Design review of the part built by this model. Coordinates are the model's own, in mm. Face numbers are marked on the shaded views. A direction names the side the tool comes from. Coordinates: 2 decimals unless noted, no trailing zeros. Loops run counter-clockwise (first coordinate to the right, second up) from the corner with the lowest first, then second, coordinate; pieces in that order, holes last. Notation, with made-up numbers: (39.5, -39.5) - (62.5, -39.5) arc R30 cw to (62.5, -0.5) - close; hole circle Ø2 at (-30.75, 88). An arc over 180 degrees is marked (long way). Use one line per item in the form item = value. Start each with the question number.
(1) Tool access review of the marked faces 4, 5 and 6: name each direction out of +Z, -Z, +X, -X, +Y, -Y from which nothing blocks a thin tool from reaching the whole face with its end or side.
(2) Add section C-C (z = -8). State the section outline as (x, y) points.
(3) Clearance check with flat-ended pins moving along their axes: pin 1 Ø13 at (x, z) = (26, -27) entering from +Y; pin 2 Ø4.5 at (x, z) = (-29, -8) entering from +Y (3 decimals); pin 3 Ø3.5 at (y, z) = (19.5, -33.5) entering from +X; pin 4 Ø5.5 at (y, z) = (20.5, -34.5) entering from -X. State where each tip first meets the part, or that it passes through.
(4) Add section D-D (y = 6). State the section outline as (x, z) points.
(5) For L1, parallel to X at y = 3, z = -29; L2, parallel to Z at x = -29, y = 2.85; L3, parallel to Y at x = 0, z = -7.5, list the stretches that pass through material, from the lowest coordinate up.
(6) Add section B-B (z = -30). State the section outline as (x, y) points.
(7) The part is to be moulded in two halves that separate along X. For the marked faces 1, 2 and 3, say which applies: pulls with the +X half, pulls with the -X half, needs draft (parallel to the pull), parting line crosses it, or undercut.
(8) Add section A-A (x = -25). State the section outline as (y, z) points.
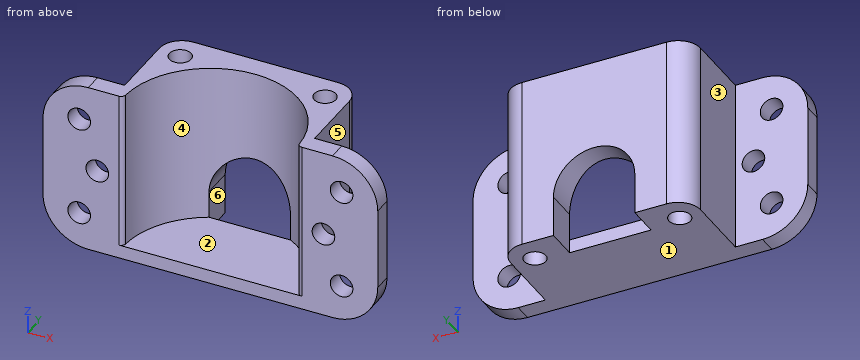
```python
from build123d import *

# Parameters (mm, degrees)
SKETCH1_W           = 42
SKETCH1_H           = 48
SKETCH1_R           = 19.25
SKETCH1_R_2         = 2.4
BOSS_EXTRUDE1_DEPTH = 35
SKETCH4_W           = 19
SKETCH4_H           = 5
BOSS_EXTRUDE3_DEPTH = 35
CUT_EXTRUDE1_REACH  = 70.367
SKETCH5_R           = 2.5
BOSS_EXTRUDE4_DEPTH = 3
CUT_EXTRUDE2_REACH  = 62.166
SKETCH9_W           = 16
SKETCH9_H           = 4
BOSS_EXTRUDE6_DEPTH = 38
CUT_EXTRUDE3_REACH  = 58.683
SKETCH10_R          = 2.5
FILLET1_R           = 10
FILLET2_R           = 5
SKETCH11_R          = 2.4
CUT_EXTRUDE4_DEPTH  = 57.302753041
FILLET3_R           = 1
CUT_EXTRUDE7_DEPTH  = 7


with BuildPart() as part:
    # Sketch1 → Boss-Extrude1 (new body)
    with BuildSketch(Plane.XY):
        Rectangle(SKETCH1_W, SKETCH1_H)
        Circle(SKETCH1_R, mode=Mode.SUBTRACT)
        with Locations((-16, 18.285714286)):
            Circle(SKETCH1_R_2, mode=Mode.SUBTRACT)
        with Locations((16, 18.285714286)):
            Circle(SKETCH1_R_2, mode=Mode.SUBTRACT)
        with Locations((16, -18.285714286)):
            Circle(SKETCH1_R_2, mode=Mode.SUBTRACT)
        with Locations((-16, -18.285714286)):
            Circle(SKETCH1_R_2, mode=Mode.SUBTRACT)
    extrude(amount=-BOSS_EXTRUDE1_DEPTH)

    # Sketch4 → Boss-Extrude3 (add)
    with BuildSketch(Plane.XY):
        with Locations((-30.5, -21.5)):
            Rectangle(SKETCH4_W, SKETCH4_H)
        with Locations((30.5, -21.5)):
            Rectangle(SKETCH4_W, SKETCH4_H)
    extrude(amount=-BOSS_EXTRUDE3_DEPTH)

    # Sketch5 → Cut-Extrude1 (cut, up to next)
    with BuildSketch(Plane(origin=(0, -19, 0), x_dir=(1, 0, 0), z_dir=(0, 1, 0)), mode=Mode.PRIVATE) as cut_extrude1_sk1:
        with Locations(Location((-25, 19, 0), (0, 0, 270))):
            Circle(SKETCH5_R)
    cut_extrude1_tool1 = extrude(cut_extrude1_sk1.sketch, amount=-CUT_EXTRUDE1_REACH, mode=Mode.PRIVATE) & part.part
    # Sketch5 → Cut-Extrude1 (cut, up to next)
    with BuildSketch(Plane(origin=(0, -19, 0), x_dir=(1, 0, 0), z_dir=(0, 1, 0)), mode=Mode.PRIVATE) as cut_extrude1_sk2:
        with Locations(Location((25, 19, 0), (0, 0, 270))):
            Circle(SKETCH5_R)
    cut_extrude1_tool2 = extrude(cut_extrude1_sk2.sketch, amount=-CUT_EXTRUDE1_REACH, mode=Mode.PRIVATE) & part.part
    add(cut_extrude1_tool1.solids().sort_by_distance((-25, -19, -19))[0], mode=Mode.SUBTRACT)
    add(cut_extrude1_tool2.solids().sort_by_distance((25, -19, -19))[0], mode=Mode.SUBTRACT)

    # Sketch6 → Boss-Extrude4 (add)
    with BuildSketch(Plane(origin=(0, 0, -35), x_dir=(-1, 0, 0), z_dir=(0, 0, -1))):
        Polygon((-21, 24), (-21, -19), (-40, -19), (-40, -24), (40, -24), (40, -19), (21, -19), (21, 24), align=None)
    extrude(amount=BOSS_EXTRUDE4_DEPTH)

    # Sketch7 → Cut-Extrude2 (cut, up to next)
    with BuildSketch(Plane.XY, mode=Mode.PRIVATE) as cut_extrude2_sk1:
        Polygon((-21, 0), (21, 0), (21, -19), (40, -19), (40, -24), (-40, -24), (-40, -19), (-21, -19), align=None)
    cut_extrude2_tool1 = extrude(cut_extrude2_sk1.sketch, amount=-CUT_EXTRUDE2_REACH, mode=Mode.PRIVATE) & part.part
    add(cut_extrude2_tool1.solids().sort_by_distance((0, -13.506678, 0))[0], mode=Mode.SUBTRACT)

    # Sketch9 → Boss-Extrude6 (add)
    with BuildSketch(Plane.XY):
        with Locations((-29, 2)):
            Rectangle(SKETCH9_W, SKETCH9_H)
        with Locations((29, 2)):
            Rectangle(SKETCH9_W, SKETCH9_H)
    extrude(amount=-BOSS_EXTRUDE6_DEPTH)

    # Sketch10 → Cut-Extrude3 (cut, up to next)
    with BuildSketch(Plane(origin=(0, 4, 0), x_dir=(1, 0, 0), z_dir=(0, 1, 0)), mode=Mode.PRIVATE) as cut_extrude3_sk1:
        with Locations(Location((-29, 8, 0), (0, 0, 180))):
            Circle(SKETCH10_R)
    cut_extrude3_tool1 = extrude(cut_extrude3_sk1.sketch, amount=-CUT_EXTRUDE3_REACH, mode=Mode.PRIVATE) & part.part
    # Sketch10 → Cut-Extrude3 (cut, up to next)
    with BuildSketch(Plane(origin=(0, 4, 0), x_dir=(1, 0, 0), z_dir=(0, 1, 0)), mode=Mode.PRIVATE) as cut_extrude3_sk2:
        with Locations(Location((-29, 30, 0), (0, 0, 180))):
            Circle(SKETCH10_R)
    cut_extrude3_tool2 = extrude(cut_extrude3_sk2.sketch, amount=-CUT_EXTRUDE3_REACH, mode=Mode.PRIVATE) & part.part
    # Sketch10 → Cut-Extrude3 (cut, up to next)
    with BuildSketch(Plane(origin=(0, 4, 0), x_dir=(1, 0, 0), z_dir=(0, 1, 0)), mode=Mode.PRIVATE) as cut_extrude3_sk3:
        with Locations(Location((29, 30, 0), (0, 0, 270))):
            Circle(SKETCH10_R)
    cut_extrude3_tool3 = extrude(cut_extrude3_sk3.sketch, amount=-CUT_EXTRUDE3_REACH, mode=Mode.PRIVATE) & part.part
    # Sketch10 → Cut-Extrude3 (cut, up to next)
    with BuildSketch(Plane(origin=(0, 4, 0), x_dir=(1, 0, 0), z_dir=(0, 1, 0)), mode=Mode.PRIVATE) as cut_extrude3_sk4:
        with Locations(Location((29, 8, 0), (0, 0, 270))):
            Circle(SKETCH10_R)
    cut_extrude3_tool4 = extrude(cut_extrude3_sk4.sketch, amount=-CUT_EXTRUDE3_REACH, mode=Mode.PRIVATE) & part.part
    # Sketch10 → Cut-Extrude3 (cut, up to next)
    with BuildSketch(Plane(origin=(0, 4, 0), x_dir=(1, 0, 0), z_dir=(0, 1, 0)), mode=Mode.PRIVATE) as cut_extrude3_sk5:
        with Locations(Location((-25, 19, 0), (0, 0, 180))):
            Circle(SKETCH10_R)
    cut_extrude3_tool5 = extrude(cut_extrude3_sk5.sketch, amount=-CUT_EXTRUDE3_REACH, mode=Mode.PRIVATE) & part.part
    # Sketch10 → Cut-Extrude3 (cut, up to next)
    with BuildSketch(Plane(origin=(0, 4, 0), x_dir=(1, 0, 0), z_dir=(0, 1, 0)), mode=Mode.PRIVATE) as cut_extrude3_sk6:
        with Locations(Location((25, 19, 0), (0, 0, 270))):
            Circle(SKETCH10_R)
    cut_extrude3_tool6 = extrude(cut_extrude3_sk6.sketch, amount=-CUT_EXTRUDE3_REACH, mode=Mode.PRIVATE) & part.part
    add(cut_extrude3_tool1.solids().sort_by_distance((-29, 4, -8))[0], mode=Mode.SUBTRACT)
    add(cut_extrude3_tool2.solids().sort_by_distance((-29, 4, -30))[0], mode=Mode.SUBTRACT)
    add(cut_extrude3_tool3.solids().sort_by_distance((29, 4, -30))[0], mode=Mode.SUBTRACT)
    add(cut_extrude3_tool4.solids().sort_by_distance((29, 4, -8))[0], mode=Mode.SUBTRACT)
    add(cut_extrude3_tool5.solids().sort_by_distance((-25, 4, -19))[0], mode=Mode.SUBTRACT)
    add(cut_extrude3_tool6.solids().sort_by_distance((25, 4, -19))[0], mode=Mode.SUBTRACT)

    # Fillet1
    fillet1_edges = [part.edges().sort_by_distance(p)[0] for p in [
        (-37, 2, 0),
        (-37, 2, -38),
        (37, 2, 0),
        (37, 2, -38),
    ]]
    fillet(fillet1_edges, radius=FILLET1_R)

    # Fillet2
    fillet2_edges = [part.edges().sort_by_distance(p)[0] for p in [
        (-21, 24, -19),
        (21, 24, -19),
    ]]
    fillet(fillet2_edges, radius=FILLET2_R)

    # Sketch11 → Cut-Extrude4 (cut, through all)
    with BuildSketch(Plane.XY.offset(-35)):
        with Locations((16, 18.285714286)):
            Circle(SKETCH11_R)
        with Locations((-16, 18.285714286)):
            Circle(SKETCH11_R)
    extrude(amount=-CUT_EXTRUDE4_DEPTH, mode=Mode.SUBTRACT)

    # Fillet3
    fillet3_edges = [part.edges().sort_by_distance(p)[0] for p in [
        (-19.25, 0, -17.5),
        (19.25, 0, -17.5),
    ]]
    fillet(fillet3_edges, radius=FILLET3_R)

    # Sketch12 → Cut-Extrude7 (cut)
    with BuildSketch(Plane(origin=(0, 24, 0), x_dir=(1, 0, 0), z_dir=(0, 1, 0))):
        with BuildLine():
            ThreePointArc((1.6e-08, 38), (-6.363961025, 35.363961036), (-9, 29))
            Line((-9, 29), (9, 29))
            ThreePointArc((9, 29), (6.363961036, 35.363961025), (1.6e-08, 38))
        make_face()
        with BuildLine():
            Line((9, 29), (-9, 29))
            ThreePointArc((-9, 29), (0, 20), (9, 29))
        make_face()
        with BuildLine():
            ThreePointArc((1.6e-08, 38), (6.363961036, 35.363961025), (9, 29))
            Line((9, 29), (9, 38))
            Line((9, 38), (1.6e-08, 38))
        make_face()
        with BuildLine():
            Line((-9, 38), (-9, 29))
            ThreePointArc((-9, 29), (-6.363961025, 35.363961036), (1.6e-08, 38))
            Line((1.6e-08, 38), (-9, 38))
        make_face()
    extrude(amount=-CUT_EXTRUDE7_DEPTH, mode=Mode.SUBTRACT)


solid = part.part
```
Computed values:
q1.face_4 = +Z, -Y
q1.face_5 = +Z, -Z, +X, +Y
q1.face_6 = -Z, +Y
q2.outline = (-36.8, 0) - (-31.5, 0) - (-31.5, 4) - (-36.8, 4) - close; (-26.5, 0) - (-20.23, 0) arc R1 ccw to (-19.23, 0.95) arc R19.25 cw to (19.23, 0.95) arc R1 ccw to (20.23, 0) - (26.5, 0) - (26.5, 4) - (21, 4) - (21, 19) arc R5 ccw to (16, 24) - (-16, 24) arc R5 ccw to (-21, 19) - (-21, 4) - (-26.5, 4) - close; (31.5, 0) - (36.8, 0) - (36.8, 4) - (31.5, 4) - close; hole circle Ø4.8 at (-16, 18.29); hole circle Ø4.8 at (16, 18.29)
q3.pin_1 = 22.57
q3.pin_2 = through
q3.pin_3 = 21
q3.pin_4 = -21
q4.outline = (-21, -38) - (21, -38) - (21, 0) - (18.29, 0) - (18.29, -35) - (-18.29, -35) - (-18.29, 0) - (-21, 0) - close
q5.L1 = -36.95 to -31.29, -26.71 to -19.01, 19.01 to 26.71, 31.29 to 36.95
q5.L2 = -37.8 to -32.5, -27.5 to -10.5, -5.5 to -0.2
q5.L3 = 19.25 to 24
q6.outline = (-36.8, 0) - (-31.5, 0) - (-31.5, 4) - (-36.8, 4) - close; (-26.5, 0) - (-20.23, 0) arc R1 ccw to (-19.23, 0.95) arc R19.25 cw to (-9, 17.02) - (-9, 24) - (-16, 24) arc R5 ccw to (-21, 19) - (-21, 4) - (-26.5, 4) - close; (9, 17.02) arc R19.25 cw to (19.23, 0.95) arc R1 ccw to (20.23, 0) - (26.5, 0) - (26.5, 4) - (21, 4) - (21, 19) arc R5 ccw to (16, 24) - (9, 24) - close; (31.5, 0) - (36.8, 0) - (36.8, 4) - (31.5, 4) - close; hole circle Ø4.8 at (-16, 18.29); hole circle Ø4.8 at (16, 18.29)
q7.face_1 = needs draft
q7.face_2 = undercut
q7.face_3 = pulls with the -X half
q8.outline = (0, -38) - (4, -38) - (4, -21.5) - (0, -21.5) - close; (0, -16.5) - (4, -16.5) - (4, 0) - (0, 0) - close
